Could you check a few things on this model? Use its own coordinates, in mm. Face numbers are marked on the shaded views. A direction names the side the tool comes from. Give positions to 0.01 mm unless a question says otherwise; leave off trailing zeros. Write each loop counter-clockwise with the first axis right and the second up, starting at its lowest first coordinate (ties: lowest second). Pieces come first, ordered by that corner, then holes. Notation, with made-up numbers: (-4.5, 18) - (14.5, 18) arc R20 ccw to (14.5, 35) - close; hole circle Ø2 at (42, 22). An arc over 180 degrees is marked (long way). Answer in a Markdown table with one row per item.
from build123d import *

# Parameters (mm, degrees)
BOSS_EXTRUDE1_DEPTH = 20
SKETCH2_W           = 5
SKETCH2_H           = 20
BOSS_EXTRUDE2_DEPTH = 5
CUT_EXTRUDE1_DEPTH  = 5
SKETCH4_W           = 5
SKETCH4_H           = 15
BOSS_EXTRUDE4_DEPTH = 5
CUT_EXTRUDE3_DEPTH  = 5
SKETCH7_W           = 5
SKETCH7_H           = 15
BOSS_EXTRUDE5_DEPTH = 5
CUT_EXTRUDE4_DEPTH  = 5
BOSS_EXTRUDE6_DEPTH = 20
CUT_EXTRUDE15_DEPTH = 61
BOSS_EXTRUDE7_DEPTH = 5
SKETCH11_W          = 5
SKETCH11_H          = 5
BOSS_EXTRUDE8_DEPTH = 5


with BuildPart() as part:
    # Sketch1 → Boss-Extrude1 (new body)
    with BuildSketch(Plane(origin=(0, 0, 0), x_dir=(1, 0, 0), z_dir=(0, 1, 0))):
        Polygon((-23.791469194, 10), (-8.791469194, 10), (-8.791469194, 0), (-13.791469194, 0), (-18.791469194, 5), (-23.791469194, 5), align=None)
    extrude(amount=BOSS_EXTRUDE1_DEPTH)

    # Sketch2 → Boss-Extrude2 (add)
    with BuildSketch(Plane.XY):
        with Locations((-11.291469194, 10)):
            Rectangle(SKETCH2_W, SKETCH2_H)
    extrude(amount=BOSS_EXTRUDE2_DEPTH)

    # Sketch3 → Cut-Extrude1 (cut)
    with BuildSketch(Plane.ZY.offset(13.791469194)):
        Polygon((0, 20), (5, 15), (5, 20), align=None)
    extrude(amount=-CUT_EXTRUDE1_DEPTH, mode=Mode.SUBTRACT)

    # Sketch4 → Boss-Extrude4 (add)
    with BuildSketch(Plane.ZY.offset(23.791469194)):
        with Locations((-7.5, 7.5)):
            Rectangle(SKETCH4_W, SKETCH4_H)
    extrude(amount=BOSS_EXTRUDE4_DEPTH)

    # Sketch6 → Cut-Extrude3 (cut)
    with BuildSketch(Plane.XY.offset(-5)):
        Polygon((-23.791469194, 15), (-28.791469194, 15), (-28.791469194, 10), align=None)
    extrude(amount=-CUT_EXTRUDE3_DEPTH, mode=Mode.SUBTRACT)

    # Sketch7 → Boss-Extrude5 (add)
    with BuildSketch(Plane.XY.offset(5)):
        with Locations((-11.291469194, 7.5)):
            Rectangle(SKETCH7_W, SKETCH7_H)
    extrude(amount=BOSS_EXTRUDE5_DEPTH)

    # Sketch8 → Cut-Extrude4 (cut)
    with BuildSketch(Plane.XY.offset(10)):
        Polygon((-8.791469194, 15), (-13.791469194, 15), (-13.791469194, 10), align=None)
    extrude(amount=-CUT_EXTRUDE4_DEPTH, mode=Mode.SUBTRACT)

    # Sketch9 → Boss-Extrude6 (add)
    with BuildSketch(Plane(origin=(0, 0, 0), x_dir=(-1, 0, 0), z_dir=(0, -1, 0))):
        Polygon((28.791469194, 5), (18.791469194, 5), (13.791469194, 0), (13.791469194, -5), (18.791469194, -5), align=None)
    extrude(amount=-BOSS_EXTRUDE6_DEPTH)

    # 3DSketch1 → Cut-Extrude15 (cut, along a direction that is not the sketch's normal)
    with BuildSketch(Plane(origin=(-28.791469194, 10, -5), x_dir=(0.8017837257372719, 0.2672612419124303, 0.5345224838248478), z_dir=(-0.5773502691896281, 0.5773502691896282, 0.5773502691896213))):
        Polygon((0, 0), (10.690449676, 9.258200998), (17.371980724, 6.943650748), (18.708286934, 0), (13.363062096, -4.629100499), align=None)
    extrude(amount=CUT_EXTRUDE15_DEPTH, dir=(0, 1, 0), mode=Mode.SUBTRACT)

    # Sketch10 → Boss-Extrude7 (add)
    with BuildSketch(Plane(origin=(0, 0, 0), x_dir=(-1, 0, 0), z_dir=(0, -1, 0))):
        Polygon((28.791469194, 5), (18.791469194, -5), (13.791469194, -5), (13.791469194, -10), (23.791469194, -10), (28.791469194, -5), align=None)
    extrude(amount=-BOSS_EXTRUDE7_DEPTH)

    # Sketch11 → Boss-Extrude8 (add)
    with BuildSketch(Plane(origin=(0, 5, 0), x_dir=(1, 0, 0), z_dir=(0, 1, 0))):
        with Locations((-16.291469194, -7.5)):
            Rectangle(SKETCH11_W, SKETCH11_H)
        Polygon((-23.791469194, -5), (-18.791469194, -5), (-23.791469194, 0), align=None)
    extrude(amount=BOSS_EXTRUDE8_DEPTH)


solid = part.part
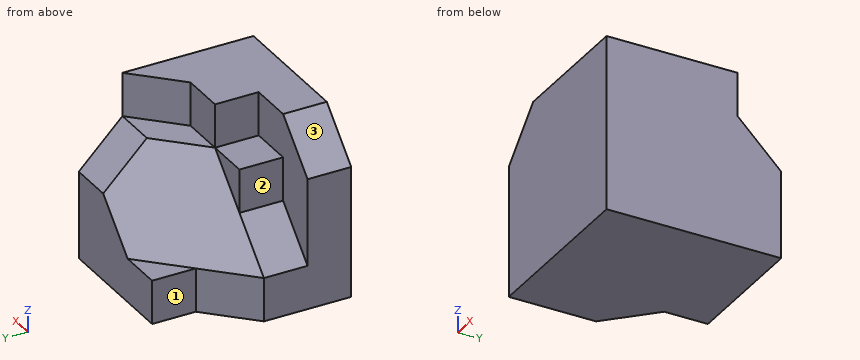
1) Imagine slicing it at C-C (x = -15.5). List the corners of the cut face in (y, z) for me.
Check values:
| item | result |
|---|---|
| outline | (0, -10) - (20, -10) - (20, -1.71) - (13.29, 5) - (10, 5) - (10, 10) - (0, 10) - close |
2) Imagine slicing it at B-B (z = -5.75). List the corners of the cut face in (x, y) for me.
Check values:
| item | result |
|---|---|
| outline | (-28.79, 0) - (-8.79, 0) - (-8.79, 20) - (-23.79, 20) - (-23.79, 15) - (-28.79, 10) - close |
3) On a 3-axis mill with a long thin cutter (end or side, diameter ignored), from which of +Z, -Z, +X, -X, +Y, -Y can I reach the whole of each face in a straight line? I mean the marked faces 1, 2 and 3. Say none if no direction works.
Check values:
| item | result |
|---|---|
| face 1 | +Z, -Z, -X, +Y |
| face 2 | +Z, -X, +Y |
| face 3 | +Z, -X, +Y, -Y |
4) Imagine slicing it at A-A (y = 9.5). List the corners of the cut face in (x, z) for me, then the cut area to 4 significant figures.
Check values:
| item | result |
|---|---|
| outline | (-28.79, -10) - (-8.79, -10) - (-8.79, 10) - (-18.79, 10) - (-18.79, 5) - (-23.79, 5) - (-23.79, 0) - (-28.79, -5) - close |
| area | 312.5 mm2 |
5) Imagine slicing it at D-D (y = 1.75). List the corners of the cut face in (x, z) for me, then the cut area to 4 significant figures.
Check values:
| item | result |
|---|---|
| outline | (-28.79, -10) - (-8.79, -10) - (-8.79, 10) - (-23.79, 10) - (-28.79, 5) - close |
| area | 387.5 mm2 |
6) Will these pins go through, and if not, where does the flat tip stop? P1, Ø4, axis at x = -20.5, y = 8, coming from the +Z side; P2, Ø5.5, axis at y = 18.5, z = -8, coming from the -X side; P3, Ø5, axis at x = -24.5, z = 4, coming from the +Y side; P4, Ø1.5, axis at x = -18.5, y = 11, coming from the +Z side.
Check values:
| item | result |
|---|---|
| P1 | stops at z = 10 |
| P2 | stops at x = -23.79 |
| P3 | stops at y = 10 |
| P4 | stops at z = 5 |
7) If I drill on line 1 (Y direction, x = -25.5, z = -0.5); line 2 (Y direction, x = -15.5, z = 8.5); line 3 (X direction, y = 8.25, z = 8), over which ranges is the centre line in solid material (lowest first)?
Check values:
| item | result |
|---|---|
| line 1 | y = 0 to 5 |
| line 2 | y = 0 to 10 |
| line 3 | x = -18.79 to -8.79 |
